Input: part model. Units: mm. Frame: model coordinates. Coordinates: 2 decimals unless noted, no trailing zeros. Write each loop counter-clockwise with the first axis right and the second up, starting at its lowest first coordinate (ties: lowest second). Pieces come first, ordered by that corner, then holes. Notation, with made-up numbers: (-11, 59.25) - (3, 59.25) arc R16 ccw to (3, 65.25) - close; hole circle Ø11 at (10.25, 66). An arc over 180 degrees is marked (long way). Use a Markdown table: item, result. Add a question column.
Q1. Section query B-B (x = 111). Return the cut outline in (y, z), then the cut area to 3 significant figures.
Q2. Pin query (flat end, axial travel): P1, Ø1, axis at x = -45.5, z = 19, coming from the -Y side; P2, Ø6, axis at x = 94, z = 22.5, coming from the +Y side; P3, Ø4, axis at y = -12, z = 57, coming from the -X side. Return the tip coordinate at first contact, or that it passes through.
Q3. Section query A-A (z = 54.5). Return the cut outline in (x, y).
Q4. Material intervals for probe 1 along Z at (x, y) = (90, -11.25); probe 2 along X at (y, z) = (-12.25, 51), sorted ascending. Write a range as from..to.
Q5. Section query C-C (y = -16.25). Give the number of separate pieces and of enclosed holes in the cut face, then the cut area to 3 significant figures.
Q6. Section query D-D (z = 25.5). Return the cut outline in (x, y), then the cut area to 3 significant figures.
from build123d import *

# Parameters (mm, degrees)
F0_W          = 254
F0_H          = 139.7
F1_DEPTH      = 19.05
F2_W          = 254
F2_H          = 19.05
F3_DEPTH      = 12.7
F4_W          = 6.35
F4_H          = 38.1
F5_DEPTH      = 12.7
F8_R          = 6.35
F9_DEPTH      = 12.7
F9_DEPTH_BACK = 12.7


with BuildPart() as f1:
    # F0 (on Front) → F1 (new body)
    with BuildSketch(Plane.XZ):
        Rectangle(F0_W, F0_H)
    extrude(amount=F1_DEPTH)

    # F2 (on face) → F3 (cut)
    with BuildSketch(Plane.XZ.offset(19.05)):
        with Locations((0, 22.225)):
            Rectangle(F2_W, F2_H)
    extrude(amount=-F3_DEPTH, mode=Mode.SUBTRACT)

    # F4 (on face) → F5 (cut)
    with BuildSketch(Plane.XZ.offset(19.05)):
        with Locations((-3.175, 50.8)):
            Rectangle(F4_W, F4_H)
        with Locations((-123.825, 50.8)):
            Rectangle(F4_W, F4_H)
    extrude(amount=-F5_DEPTH, mode=Mode.SUBTRACT)

    # F8 (on face) → F9 (cut, two sides)
    with BuildSketch(Plane(origin=(0, 5.1184025608, -3.5839440567), x_dir=(-1, 0, 0), z_dir=(0, 0.8191520443, -0.5735764364))) as f9_sk:
        with Locations((76.2, -42.1363239999)):
            Circle(F8_R)
    extrude(amount=F9_DEPTH, mode=Mode.SUBTRACT)
    extrude(f9_sk.sketch, amount=-F9_DEPTH_BACK, mode=Mode.SUBTRACT)


solid = f1.part
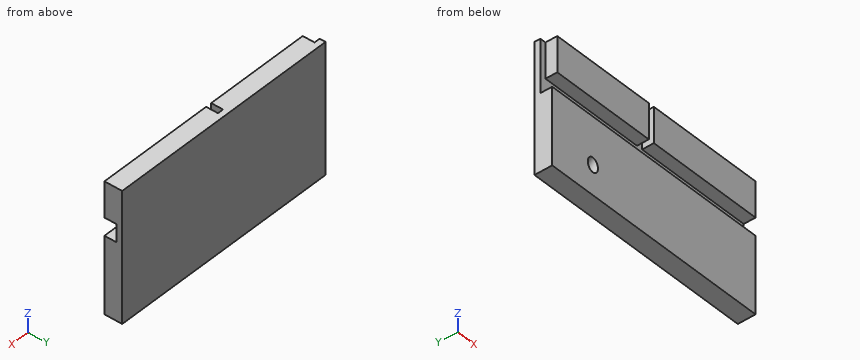
Values follow:
| question | item | result |
|---|---|---|
| 1 | outline | (-19.05, -69.85) - (0, -69.85) - (0, 69.85) - (-19.05, 69.85) - (-19.05, 31.75) - (-6.35, 31.75) - (-6.35, 12.7) - (-19.05, 12.7) - close |
| 1 | area | 2,420 mm2 |
| 2 | P1 | y = -6.35 |
| 2 | P2 | y = 0 |
| 2 | P3 | x = -120.65 |
| 3 | outline | (-127, -6.35) - (-120.65, -6.35) - (-120.65, -19.05) - (-6.35, -19.05) - (-6.35, -6.35) - (0, -6.35) - (0, -19.05) - (127, -19.05) - (127, 0) - (-127, 0) - close |
| 4 | probe 1 | -69.85..12.7, 31.75..69.85 |
| 4 | probe 2 | -120.65..-6.35, 0..127 |
| 5 | separate pieces | 3 |
| 5 | enclosed holes | 1 |
| 5 | area | 30,000 mm2 |
| 6 | outline | (-127, -6.35) - (127, -6.35) - (127, 0) - (-127, 0) - close |
| 6 | area | 1,610 mm2 |
